```python
from build123d import *

# Parameters (mm, degrees)
F1_DEPTH    = 3.65
F2_T        = -1
F3_T1_DEPTH = 7.0190808226
F3_T3_DEPTH = 12.2237754854
F3_T6_ANGLE = 180
F3_T8_ANGLE = 180


# Not quite as in the source:
# - a fillet or chamfer that OpenCascade refuses, or shapes differently, is made with other operations: its cross-section is extruded or revolved along the edge and cut away or added


with BuildPart() as f1:
    # F0 (on Top) → F1 (new body)
    with BuildSketch(Plane.XY):
        with BuildLine():
            ThreePointArc((-2.5, 10.9379339914), (-6.9942261902, -8.773209219), (11.22, 0))
            ThreePointArc((11.22, 0), (8.773209219, 6.9942261902), (2.5, 10.9379339914))
            Line((2.5, 10.9379339914), (2.5, 0))
            ThreePointArc((2.5, 0), (0, -2.5), (-2.5, 0))
            Line((-2.5, 0), (-2.5, 10.9379339914))
        make_face()
    extrude(amount=F1_DEPTH)

    # F2
    f2_openings = [f1.faces().sort_by_distance(p)[0] for p in [
        (-6.797639, -8.52662, 3.65),
    ]]
    offset(amount=F2_T, openings=f2_openings)

    # F3: chamfer of 0.5 on 8 edges, made by hand

    # F3_s2 → F3_t1 (cut)
    with BuildSketch(Plane.XY.offset(-1.6845404113)):
        with BuildLine():
            Line((-3.1399253731, 10.7716882916), (-2.5, 10.2916665317))
            Line((-2.5, 10.2916665317), (-2.5, 10.9379339914))
            ThreePointArc((-2.5, 10.9379339914), (-2.8272189257, 10.857957135), (-3.1399253731, 10.7716882916))
        make_face()
        with BuildLine():
            Line((3.1399253731, 10.7716882916), (2.5, 10.2916665317))
            Line((2.5, 10.2916665317), (2.5, 10.9379339914))
            ThreePointArc((2.5, 10.9379339914), (2.8272189257, 10.857957135), (3.1399253731, 10.7716882916))
        make_face()
    extrude(amount=F3_T1_DEPTH, mode=Mode.SUBTRACT)

    # F3_s4 → F3_t3 (cut)
    with BuildSketch(Plane.XZ.offset(-12.2237754854)):
        Polygon((2.5, 0.5), (3, 0), (2.5, 0), align=None)
        Polygon((2.5, 3.15), (3, 3.65), (2.5, 3.65), align=None)
        Polygon((-2.5, 0.5), (-3, 0), (-2.5, 0), align=None)
        Polygon((-2.5, 3.15), (-3, 3.65), (-2.5, 3.65), align=None)
    extrude(amount=F3_T3_DEPTH, mode=Mode.SUBTRACT)

    # F3_s5 → F3_t6 (revolve, cut)
    with BuildSketch(Plane.XZ):
        Polygon((2.5, 3.15), (3, 3.65), (2.5, 3.65), align=None)
    revolve(axis=Axis((0, 0, 3.65), (0, 0, -1)), revolution_arc=F3_T6_ANGLE, mode=Mode.SUBTRACT)

    # F3_s7 → F3_t8 (revolve, cut)
    with BuildSketch(Plane.XZ):
        Polygon((2.5, 0.5), (3, 0), (2.5, 0), align=None)
    revolve(axis=Axis((0, 0, 0), (0, 0, -1)), revolution_arc=F3_T8_ANGLE, mode=Mode.SUBTRACT)


solid = f1.part
```
Design review of the part built by this model. Coordinates are the model's own, in mm. A direction names the side the tool comes from. Round coordinates to 2 decimals unless told otherwise and drop trailing zeros. Write each loop counter-clockwise with the first axis right and the second up, starting at its lowest first coordinate (ties: lowest second). Pieces come first, ordered by that corner, then holes. Notation, with made-up numbers: (44, 59.25) -> (49, 59.25) arc R11 cw to (49, 75.25) -> close; hole circle Ø1 at (68.25, 43). An arc over 180 degrees is marked (long way). Write item = value, one per line. Start each with the question number.
1) Take a section at B-B, the plane y = 2.75. State the section outline as (x, z) points, plus the area to 3 significant figures.
2) Take a section at C-C, the plane x = 0. State the section outline as (y, z) points.
3) Tool access review of faces 4 (the face through (2, -3, 0)), 5 (the face through (-3.5, 5, 2)), 6 (the face through (-2.5, 5, 2)): name each direction out of +Z, -Z, +X, -X, +Y, -Y from which nothing blocks a thin tool from reaching the whole face with its end or side.
4) Clearance check with flat-ended pins moving along their axes: pin 1 (1.5 mm diameter, centred on y = -4, z = 0.5, fed in from +X); pin 2 (1.5 mm diameter, centred on y = 3, z = 2, fed in from -X); pin 3 (0.8 mm diameter, centred on y = 4, z = 2.5, fed in from +X). State where each tip first meets the part, or that it passes through.
5) Wall thickness on probe 1 along X at (y, z) = (0, 2.8); probe 2 along X at (y, z) = (7.5, 3.4); probe 3 along Y at (x, z) = (0, 1.9): over which ranges is each line inside the solid? List them lowest first. Write a range as from..to.
6) Mouldability with a two-part tool opening along X and no side actions: class faces 1 (the face through (-0.45, -11.21, 1.8)), 2 (the face through (3.3, 0.6, 3.65)), 3 (the face through (0.1, -3.5, 2.3)) as +X half, -X half, draft (parallel to the pull), parting line (faces both ways), or undercut.
7) Take a section at A-A, the plane z = 2.45. State the section outline as (x, y) points, plus the area to 3 significant figures.
8) Take a section at D-D, the plane y = -8.5. State the section outline as (x, z) points.
Results list:
q1.outline = (-10.88, 0) -> (-3, 0) -> (-2.5, 0.5) -> (-2.5, 3.15) -> (-3, 3.65) -> (-3.5, 3.65) -> (-3.5, 1) -> (-9.84, 1) -> (-9.84, 3.65) -> (-10.88, 3.65) -> close; (2.5, 0.5) -> (3, 0) -> (10.88, 0) -> (10.88, 3.65) -> (9.84, 3.65) -> (9.84, 1) -> (3.5, 1) -> (3.5, 3.65) -> (3, 3.65) -> (2.5, 3.15) -> close
q1.area = 27.0 mm²
q2.outline = (-11.22, 0) -> (-3, 0) -> (-2.5, 0.5) -> (-2.5, 3.15) -> (-3, 3.65) -> (-3.5, 3.65) -> (-3.5, 1) -> (-10.22, 1) -> (-10.22, 3.65) -> (-11.22, 3.65) -> close
q3.face_4 = -Z, +X, -X, +Y, -Y
q3.face_5 = +Z
q3.face_6 = +Z, -Z, +Y
q4.pin_1 = 10.74
q4.pin_2 = -10.99
q4.pin_3 = 10.63
q5.probe_1 = -11.22..-10.22, -3.5..-2.5, 2.5..3.5, 10.22..11.22
q5.probe_2 = -8.34..-6.94, -3.5..-2.75, 2.75..3.5, 6.94..8.34
q5.probe_3 = -11.22..-10.22, -3.5..-2.5
q6.face_1 = parting line
q6.face_2 = draft
q6.face_3 = undercut
q7.outline = (-3.14, 10.77) arc R11.22 ccw (long way) to (3.14, 10.77) -> (2.5, 10.29) -> (2.5, 0) arc R2.5 cw to (-2.5, 0) -> (-2.5, 10.29) -> close; hole (-3.5, 0) -> (-3.5, 9.6) arc R10.22 ccw (long way) to (3.5, 9.6) -> (3.5, 0) arc R3.5 cw to start
q7.area = 90.8 mm²
q8.outline = (-7.32, 0) -> (7.32, 0) -> (7.32, 3.65) -> (5.67, 3.65) -> (5.67, 1) -> (-5.67, 1) -> (-5.67, 3.65) -> (-7.32, 3.65) -> close
